The listing builds one solid part. Answer for the finished solid, in the listing's coordinates (mm). A direction names the side the tool comes from. Coordinates: 2 decimals unless noted, no trailing zeros. Loops run counter-clockwise (first coordinate to the right, second up) from the corner with the lowest first, then second, coordinate; pieces in that order, holes last. Notation, with made-up numbers: (54.25, 49.25) -> (60.25, 49.25) arc R13 ccw to (60.25, 55.25) -> close; hole circle Ø1 at (-17, 86.25). An arc over 180 degrees is marked (long way). Answer in a Markdown table with one row per item.
```python
from build123d import *

# Parameters (mm, degrees)
SKETCH1_W               = 8
SKETCH1_H               = 8
BOSS_EXTRUDE1_DEPTH     = 3
CUT_EXTRUDE1_DEPTH      = 12.704699911
CUT_EXTRUDE1_DEPTH_BACK = 12.704699911
CUT_EXTRUDE2_DEPTH      = 11
SKETCH4_R               = 1.8
CUT_EXTRUDE3_DEPTH      = 0.8
SKETCH5_W               = 8
SKETCH5_H               = 1
BOSS_EXTRUDE2_DEPTH     = 2
FILLET1_R               = 4
CUT_EXTRUDE4_DEPTH      = 0.4
CUT_EXTRUDE5_DEPTH      = 0.4


with BuildPart() as part:
    # Sketch1 → Boss-Extrude1 (new body)
    with BuildSketch(Plane(origin=(0, 0, 0), x_dir=(1, 0, 0), z_dir=(0, 1, 0))):
        with Locations((4, 4)):
            Rectangle(SKETCH1_W, SKETCH1_H)
    extrude(amount=BOSS_EXTRUDE1_DEPTH)

    # Sketch2 → Cut-Extrude1 (cut, two sides: drawn at the far end of the back side and taken through both)
    with BuildSketch(Plane.XY.offset(-CUT_EXTRUDE1_DEPTH_BACK)):
        Polygon((0, 0), (0.6, 3), (0, 3), align=None)
        Polygon((8, 0), (7.4, 3), (8, 3), align=None)
    extrude(amount=CUT_EXTRUDE1_DEPTH + CUT_EXTRUDE1_DEPTH_BACK, mode=Mode.SUBTRACT)

    # Sketch3 → Cut-Extrude2 (cut)
    with BuildSketch(Plane(origin=(0, 0, 0), x_dir=(0, 0, -1), z_dir=(1, 0, 0))):
        Polygon((0, 0), (0.6, 3), (0, 3), align=None)
        Polygon((8, 3), (7.4, 3), (8, 0), align=None)
    extrude(amount=CUT_EXTRUDE2_DEPTH, mode=Mode.SUBTRACT)

    # Sketch4 → Cut-Extrude3 (cut)
    with BuildSketch(Plane.XZ):
        with Locations(Location((4, -3.75, 0), (0, 0, 270))):
            Circle(SKETCH4_R)
    extrude(amount=-CUT_EXTRUDE3_DEPTH, mode=Mode.SUBTRACT)

    # Sketch5 → Boss-Extrude2 (add)
    with BuildSketch(Plane.XZ):
        with Locations((4, -7.5)):
            Rectangle(SKETCH5_W, SKETCH5_H)
    extrude(amount=BOSS_EXTRUDE2_DEPTH)

    # Fillet1
    # the kernel refuses this fillet: 4 mm, written as the material it takes off along each edge
    with BuildSketch(Plane(origin=(8, -2, -16.660254038), x_dir=(0, 1, 0), z_dir=(0, 0, 1)), Plane(origin=(0, -2, 1.660254038), x_dir=(0, 1, 0), z_dir=(0, 0, -1))) as fillet1_piece_1:
        with BuildLine():
            CenterArc((4, 3.464101615), FILLET1_R, 180, 60)
            Line((0, 3.464101615), (-0.08, 3.464101615))
            Line((-0.08, 3.464101615), (-0.08, 0))
            Line((-0.08, 0), (0, -0.08))
            ThreePointArc((0, -0.08), (1, -0.08), (1.96, -0.069282032))
            Line((1.96, -0.069282032), (2, 0))
        make_face()
    extrude(amount=18.320508076, mode=Mode.SUBTRACT)

    # Sketch6 → Cut-Extrude4 (cut)
    with BuildSketch(Plane(origin=(0, 3, 0), x_dir=(1, 0, 0), z_dir=(0, 1, 0))):
        with BuildLine():
            Line((2.312898911, 2.041410717), (2.312898911, 6.041410717))
            Line((2.312898911, 6.041410717), (3.991584808, 6.041410717))
            add(Edge.make_bspline(
                [(3.991584808, 6.041410717), (4.042601732, 6.041096301), (4.140920681, 6.040490364), (4.283109063, 6.036071747), (4.414238667, 6.026814487), (4.534891188, 6.016330564), (4.644487122, 6.001077132), (4.74345979, 5.982803671), (4.831642566, 5.961627249), (4.910322089, 5.936265049), (4.982061831, 5.90723713), (5.04889092, 5.87268574), (5.111544162, 5.83220454), (5.170983849, 5.787188805), (5.227461685, 5.737569368), (5.279429347, 5.682033053), (5.32779225, 5.621406813), (5.372511371, 5.556195062), (5.411906117, 5.48668575), (5.447902572, 5.415111184), (5.477205044, 5.340709703), (5.50140862, 5.263831792), (5.52074281, 5.184644366), (5.534162371, 5.102946099), (5.542540058, 5.018884869), (5.543287935, 4.962103945), (5.543668142, 4.93323764)],
                knots=[0, 0, 0, 0, 1.675828044, 3.229627355, 4.67171229, 5.993455049, 7.206927059, 8.304770529, 9.29850117, 10.183580433, 11.017754134, 11.837875825, 12.650738409, 13.464925643, 14.285328857, 15.117007378, 15.959673368, 16.830859064, 17.711229498, 18.58228265, 19.460420693, 20.334473227, 21.228207035, 22.135446768, 23.052097822, 24, 24, 24, 24], degree=3))
            add(Edge.make_bspline(
                [(5.543668142, 4.93323764), (5.542962916, 4.896874176), (5.541584712, 4.825809944), (5.528901745, 4.721651895), (5.5100643, 4.622136315), (5.483211668, 4.527125334), (5.446289845, 4.437736414), (5.403428122, 4.352717347), (5.352308317, 4.272356517), (5.293277733, 4.19745058), (5.226389218, 4.127933229), (5.151349641, 4.065235076), (5.06869476, 4.009111084), (4.977924564, 3.959884897), (4.879671091, 3.917801842), (4.77350828, 3.882394441), (4.659916733, 3.853576761), (4.580902516, 3.840017181), (4.540463013, 3.833077384)],
                knots=[0, 0, 0, 0, 1.05911256, 2.069797862, 3.05271628, 4.008392045, 4.940519534, 5.866323021, 6.779546087, 7.71056835, 8.640711998, 9.585328432, 10.554502533, 11.547017206, 12.589327225, 13.664782803, 14.804835066, 16, 16, 16, 16], degree=3))
            add(Edge.make_bspline(
                [(4.540463013, 3.833077384), (4.579572554, 3.807174767), (4.656115253, 3.756479818), (4.762017587, 3.672984601), (4.857092756, 3.585349912), (4.929078878, 3.507419696), (4.984392794, 3.438888442), (5.028929947, 3.378950347), (5.076970406, 3.309970293), (5.128042999, 3.231910907), (5.183657562, 3.145462828), (5.241745689, 3.049302835), (5.303522957, 2.944368887), (5.345058377, 2.871067212), (5.366584808, 2.833077384)],
                knots=[0, 0, 0, 0, 1.285445069, 2.515791127, 3.691898215, 4.826622834, 5.420063933, 6.105349801, 6.873086501, 7.723915395, 8.66222816, 9.690593598, 10.803111229, 12, 12, 12, 12], degree=3))
            Line((5.366584808, 2.833077384), (5.851360449, 2.041410717))
            Line((5.851360449, 2.041410717), (4.952321988, 2.041410717))
            Line((4.952321988, 2.041410717), (4.383411731, 2.949263281))
            add(Edge.make_bspline(
                [(4.383411731, 2.949263281), (4.357283981, 2.985622121), (4.307400733, 3.055038622), (4.235391184, 3.153681722), (4.169508837, 3.241491798), (4.111507042, 3.319740728), (4.058450932, 3.386209972), (4.011951502, 3.442057857), (3.972955886, 3.488482798), (3.928832249, 3.534515131), (3.877499082, 3.581823547), (3.813952721, 3.627691749), (3.748696505, 3.664257396), (3.678779681, 3.692157844), (3.597922987, 3.71161189), (3.500720436, 3.724006591), (3.384115753, 3.733151261), (3.299833928, 3.733519777), (3.254405321, 3.73371841)],
                knots=[0, 0, 0, 0, 1.465447777, 2.797841088, 3.997266218, 5.05856206, 5.985598736, 6.780315439, 7.437430484, 7.969193402, 8.866571936, 9.718200644, 10.52825214, 11.309096006, 12.174169268, 13.242355782, 14.513606761, 16, 16, 16, 16], degree=3))
            Line((3.254405321, 3.73371841), (3.08212968, 3.73371841))
            Line((3.08212968, 3.73371841), (3.08212968, 2.041410717))
            Line((3.08212968, 2.041410717), (2.312898911, 2.041410717))
        make_face()
        with BuildLine():
            Line((3.08212968, 4.400385076), (3.701520706, 4.400385076))
            add(Edge.make_bspline(
                [(3.701520706, 4.400385076), (3.749332843, 4.400487541), (3.840423044, 4.400682752), (3.969955122, 4.403510317), (4.085670885, 4.405910235), (4.186877859, 4.411940131), (4.274028855, 4.417916326), (4.346774263, 4.425683211), (4.405726987, 4.434863419), (4.464610849, 4.449136231), (4.52492793, 4.474003789), (4.589214527, 4.509422512), (4.644158691, 4.555370201), (4.691753027, 4.608490376), (4.728060837, 4.670937972), (4.756498441, 4.739930879), (4.770916908, 4.817002181), (4.773239296, 4.87042263), (4.774437372, 4.89798123)],
                knots=[0, 0, 0, 0, 1.697953026, 3.23488743, 4.60134403, 5.807846676, 6.835100678, 7.703488618, 8.405232423, 8.952775585, 9.851109663, 10.713519226, 11.549115941, 12.382556273, 13.233359028, 14.101746968, 15.020727134, 16, 16, 16, 16], degree=3))
            add(Edge.make_bspline(
                [(4.774437372, 4.89798123), (4.773074786, 4.928811222), (4.770445895, 4.98829272), (4.749714088, 5.072935459), (4.713527564, 5.147705664), (4.663829732, 5.212726785), (4.601441933, 5.267631557), (4.527131165, 5.311213996), (4.441449505, 5.343672387), (4.379650359, 5.355659208), (4.347354039, 5.361923538)],
                knots=[0, 0, 0, 0, 1.062977961, 2.050844577, 2.982300261, 3.90936959, 4.856017476, 5.831122378, 6.86654153, 8, 8, 8, 8], degree=3))
            add(Edge.make_bspline(
                [(4.347354039, 5.361923538), (4.336678458, 5.363096555), (4.311375089, 5.365876852), (4.266692338, 5.367662514), (4.20955971, 5.370407271), (4.139285669, 5.371528992), (4.056498042, 5.373495271), (3.960867626, 5.373856329), (3.852698247, 5.375009885), (3.776307493, 5.374835906), (3.735975834, 5.374744051)],
                knots=[0, 0, 0, 0, 0.42127143, 0.998501726, 1.753681744, 2.66564073, 3.755712164, 5.002818897, 6.417592707, 8, 8, 8, 8], degree=3))
            Line((3.735975834, 5.374744051), (3.08212968, 5.374744051))
            Line((3.08212968, 5.374744051), (3.08212968, 4.400385076))
        make_face(mode=Mode.SUBTRACT)
    extrude(amount=-CUT_EXTRUDE4_DEPTH, mode=Mode.SUBTRACT)

    # Sketch7 → Cut-Extrude5 (cut)
    with BuildSketch(Plane(origin=(0, 3, 0), x_dir=(1, 0, 0), z_dir=(0, 1, 0))):
        Polygon((6.546707708, 0.907912363), (6.546707708, 1.256630312), (5.871066683, 1.256630312), (5.871066683, 1.53894201), (6.589956907, 2.586117491), (6.873630785, 2.586117491), (6.873630785, 1.539963645), (7.091579503, 1.539963645), (7.091579503, 1.256630312), (6.873630785, 1.256630312), (6.873630785, 0.907912363), align=None)
        Polygon((6.546707708, 1.539963645), (6.546707708, 2.105949222), (6.157805465, 1.539963645), align=None, mode=Mode.SUBTRACT)
    extrude(amount=-CUT_EXTRUDE5_DEPTH, mode=Mode.SUBTRACT)


solid = part.part
```
Item 1: Determine the mould class of faces 1 (the face through (4.541, 0.394, -5.467)), 2 (the face through (4, -1, -7)), 3 (the face through (4, 3, -3)) for opening direction Z: +Z half, -Z half, draft (parallel to the pull), parting line (faces both ways), or undercut.
Findings below:
| item | result |
|---|---|
| face 1 | undercut |
| face 2 | +Z half |
| face 3 | draft |
Item 2: A cutting plane is placed at A-A, the plane y = 0.5. Determine the outline of the cut face in (x, z), plus the area to 3 significant figures.
Findings below:
| item | result |
|---|---|
| outline | (0.1, -7.9) -> (7.9, -7.9) -> (7.9, -0.1) -> (0.1, -0.1) -> close; hole circle Ø3.6 at (4, -3.75) |
| area | 50.7 mm2 |
Item 3: Flat-ended cylindrical pins translate along their axes: pin 1 Ø2 at (x, y) = (5, -0.5) entering from +Z; pin 2 Ø1.5 at (x, z) = (7, -7) entering from -Y; pin 3 Ø4 at (x, z) = (3, -4) entering from -Y; pin 4 Ø3 at (y, z) = (2.5, -1.5) entering from +X. Find the tip coordinate at first contact, or state that the pin passes through.
Findings below:
| item | result |
|---|---|
| pin 1 | stops at z = 0 |
| pin 2 | stops at y = -1.61 |
| pin 3 | stops at y = 0 |
| pin 4 | stops at x = 7.8 |
Item 4: A tool of negligible diameter and unlimited length cuts with its end or side. For faces 4 (the face through (4, 0.8, -4)), 5 (the face through (7.7, 1.5, -4.1)), 6 (the face through (4, 2.6, -4)), 7 (the face through (3, 0, -2)), from which of +Z, -Z, +X, -X, +Y, -Y can it reach the whole face along a straight path? Write none if from no direction.
Findings below:
| item | result |
|---|---|
| face 4 | -Y |
| face 5 | +Z, -Z, +X, +Y |
| face 6 | +Y |
| face 7 | +Z, +X, -X, -Y |
Item 5: Find the intervals of material crossed by probe 1 along Y at (x, z) = (4.75, -6.75); probe 2 along Z at (x, y) = (4.25, -1.7); probe 3 along X at (y, z) = (0.4, -3.75), in increasing order.
Findings below:
| item | result |
|---|---|
| probe 1 | y = 0 to 3 |
| probe 2 | z = -8 to -7 |
| probe 3 | x = 0.08 to 2.2, 5.8 to 7.92 |
Item 6: A cutting plane is placed at C-C, the plane y = -1. Determine the outline of the cut face in (x, z), plus the area to 3 significant figures.
Findings below:
| item | result |
|---|---|
| outline | (0.82, -8) -> (7.18, -8) -> (7.18, -7) -> (0.82, -7) -> close |
| area | 6.36 mm2 |
Item 7: A cutting plane is placed at B-B, the plane x = 0.5. Determine the outline of the cut face in (y, z).
Findings below:
| item | result |
|---|---|
| outline | (-0.69, -8) -> (0, -8) -> (2.5, -7.5) -> (2.5, -0.5) -> (0, 0) -> (0, -7) -> (-0.69, -7) -> close |
